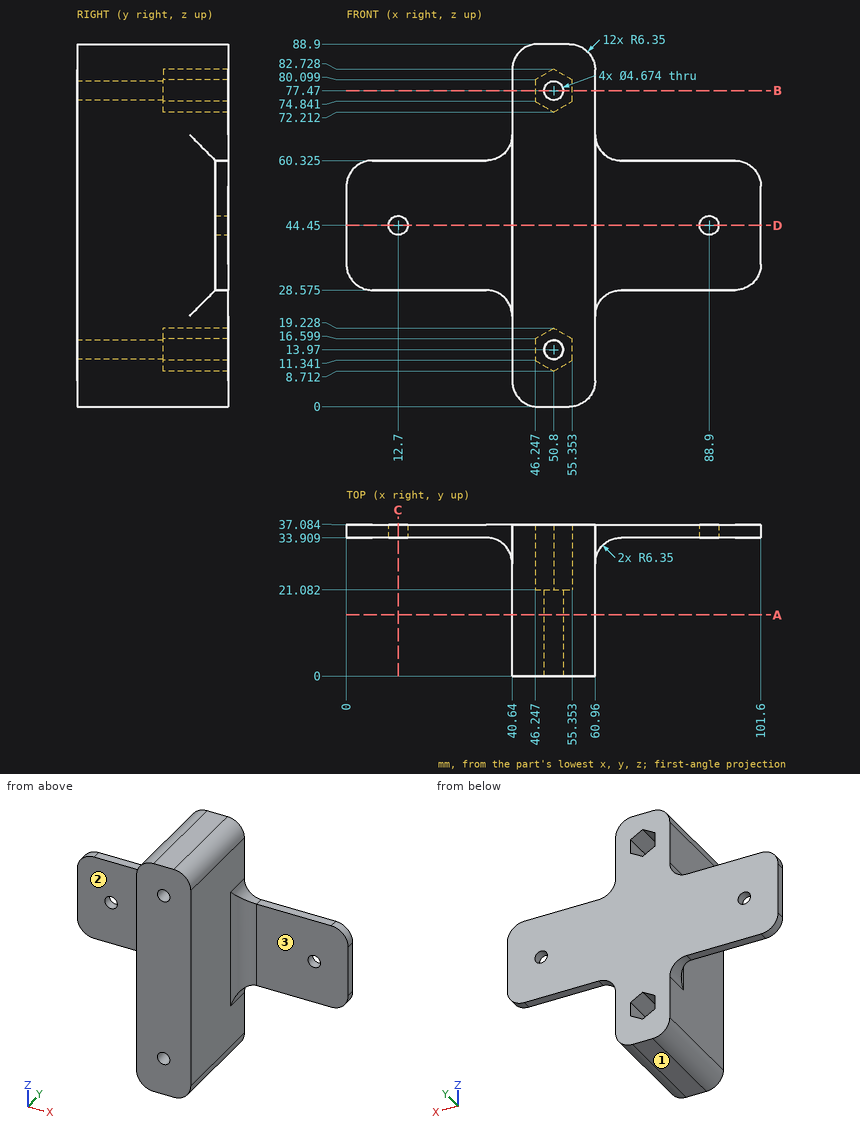
Can you work these out from the drawing? Everything is in mm from the part's minimum corner. A direction names the side the tool comes from. Round coordinates to 2 decimals unless told otherwise and drop trailing zeros. Order: outer loops, then holes, each group sorted by start corner. A loop starts at its lowest first (then second) coordinate and runs counter-clockwise, first axis right, second up.
(1) If we section it at C-C (x = 12.7): Please give me the cut outline in (y, z) (1 decimal).
Results are:
outline: (33.9, 28.6) - (37.1, 28.6) - (37.1, 42.1) - (33.9, 42.1) - close; (33.9, 46.8) - (37.1, 46.8) - (37.1, 60.3) - (33.9, 60.3) - close
(2) If I drill on L1, parallel to Z at x = 50.8, y = 14.25; L2, parallel to X at y = 11.25, z = 13.97; L3, parallel to Z at x = 49.5, y = 6.5, over which ranges is the centre line in solid material (lowest first)?
Results are:
L1: z = 0 to 11.63, 16.31 to 75.13, 79.81 to 88.9
L2: x = 40.64 to 48.46, 53.14 to 60.96
L3: z = 0 to 12.03, 15.91 to 75.53, 79.41 to 88.9
(3) If we section it at A-A (y = 15): Please give me the cut outline in (x, z).
Results are:
outline: (40.64, 6.35) arc R6.35 ccw to (46.99, 0) - (54.61, 0) arc R6.35 ccw to (60.96, 6.35) - (60.96, 82.55) arc R6.35 ccw to (54.61, 88.9) - (46.99, 88.9) arc R6.35 ccw to (40.64, 82.55) - close; hole circle Ø4.67 at (50.8, 13.97); hole circle Ø4.67 at (50.8, 77.47)
(4) On a 3-axis mill with a long thin cutter (end or side, diameter ignored), from which of +Z, -Z, +X, -X, +Y, -Y can I reach the whole of each face in a straight line? I mean the marked faces 1, 2 and 3. Say none if no direction works.
Results are:
face 1: -Z, +X, -X, +Y, -Y
face 2: +Z, -Z, -X, -Y
face 3: +Z, -Z, +X, -Y
(5) If we section it at D-D (z = 44.45): Please give me the cut outline in (x, y), plus the area to 3 significant figures.
Results are:
outline: (0, 33.91) - (10.36, 33.91) - (10.36, 37.08) - (0, 37.08) - close; (15.04, 33.91) - (34.29, 33.91) arc R6.35 cw to (40.64, 27.56) - (40.64, 0) - (60.96, 0) - (60.96, 27.56) arc R6.35 cw to (67.31, 33.91) - (86.56, 33.91) - (86.56, 37.08) - (15.04, 37.08) - close; (91.24, 33.91) - (101.6, 33.91) - (101.6, 37.08) - (91.24, 37.08) - close
area: 999 mm2
(6) I'm going to push flat-ended pins straight in: pin 1 (4 mm diameter, centred on y = 29, z = 13.5, fed in from -X); pin 2 (1.6 mm diameter, centred on y = 28.5, z = 15, fed in from +X); pin 3 (4 mm diameter, centred on x = 64.5, y = 15, fed in from +Z); pin 4 (1.6 mm diameter, centred on x = 78.5, y = 35.5, fed in from -Z) (3 decimals). Where does each tip first touch, or does it pass through?
Results are:
pin 1: stops at x = 40.64
pin 2: stops at x = 60.96
pin 3: passes through
pin 4: stops at z = 28.575
(7) If we section it at B-B (z = 77.47): Please give me the cut outline in (x, y), plus the area to 3 significant figures.
Results are:
outline: (40.64, 0) - (48.46, 0) - (48.46, 21.08) - (46.25, 21.08) - (46.25, 37.08) - (40.64, 37.08) - close; (53.14, 0) - (60.96, 0) - (60.96, 37.08) - (55.35, 37.08) - (55.35, 21.08) - (53.14, 21.08) - close
area: 509 mm2
